from build123d import *

# Parameters (mm, degrees)
BOX001_W               = 70.7107
BOX001_H               = 70.7107
BOX001_DEPTH           = 10
BOX001_PLACEMENT_ANGLE = 315
BOX002_W               = 100
BOX002_H               = 100
BOX002_DEPTH           = 20
BOX_W                  = 200
BOX_H                  = 100
BOX_DEPTH              = 50


with BuildPart() as cube001:
    # Box001 → Box001 (new body)
    with BuildSketch(Plane.XY):
        with Locations((35.35535, 35.35535)):
            Rectangle(BOX001_W, BOX001_H)
    extrude(amount=BOX001_DEPTH)


with BuildPart() as cube001_1:
    # Box001 placement: moved
    add(cube001.part.moved(Location((-50, 0, 40))).rotate(Axis((-50, 0, 40), (0, 0, 1)), BOX001_PLACEMENT_ANGLE))


with BuildPart() as cube002:
    # Box002 → Box002 (new body)
    with BuildSketch(Plane(origin=(0, -50, 10), x_dir=(1, 0, 0), z_dir=(0, 0, 1))):
        with Locations((50, 50)):
            Rectangle(BOX002_W, BOX002_H)
    extrude(amount=BOX002_DEPTH)


with BuildPart() as fusion:
    # Box → Box (new body)
    with BuildSketch(Plane(origin=(0, 50, 0), x_dir=(-1, 0, 0), z_dir=(0, 0, 1))):
        with Locations((100, 50)):
            Rectangle(BOX_W, BOX_H)
    extrude(amount=BOX_DEPTH)

    # Fusion: union Cube001, Cube002
    add(cube001_1.part)
    add(cube002.part)


solid = fusion.part
Model file for the job. Use its own axes, mm. A direction names the side the tool comes from. Give positions to 0.01 mm unless a question says otherwise; leave off trailing zeros. Loops run counter-clockwise (first coordinate to the right, second up) from the corner with the lowest first, then second, coordinate; pieces in that order, holes last. Notation, with made-up numbers: (87.25, 19.25) -> (123.25, 19.25) arc R37 ccw to (123.25, 57.25) -> close; hole circle Ø10 at (-24.5, -28). An arc over 180 degrees is marked (long way). Use a Markdown table: item, result. Add a question column.
(1) Slice it at C-C on x = 56.5. List the corners of the cut face in (y, z).
(2) Wall check: line 1 along Z through (x, y) = (25, 16); line 2 along X through (y, z) = (3, 6); line 3 along Z through (x, y) = (83.5, -26). Give the ranges that are in metal, low to high.
(3) Mould opens along Z. For faces 1 (the flat face through (49, 1, 10)), 2 (the flat face through (100, -1, 20)), 3 (the flat face through (0, 1, 35)) say: +Z half, -Z half, draft (parallel to the pull), parting line (faces both ways), or undercut.
(4) Slice it at A-A on x = 22.5. List the corners of the cut face in (y, z).
(5) Slice it at D-D on y = -7. List the corners of the cut face in (x, z).
(6) Slice it at B-B on y = 6.5. List the corners of the cut face in (x, z), and give its area (3 significant figures).
(7) Drop flat-ended pins along their axis: pin 1 Ø5 at (y, z) = (-0.5, 37) entering from +X; pin 2 Ø1 at (x, y) = (44, 18) entering from +Z; pin 3 Ø15 at (x, y) = (15, 4) entering from -Z. Give the stop position or say it passes through.
(8) Tool access for faces 4 (the flat face through (49, 1, 30)), 5 (the flat face through (0, 1, 5)), 6 (the flat face through (25, -25, 45)): list every direction of +Z, -Z, +X, -X, +Y, -Y with a clear straight run to the whole face (end or side of a thin tool).
Filled sheet:
| question | item | result |
|---|---|---|
| 1 | outline | (-50, 10) -> (50, 10) -> (50, 30) -> (-50, 30) -> close |
| 2 | line 1 | 10 to 30, 40 to 50 |
| 2 | line 2 | -200 to 0 |
| 2 | line 3 | 10 to 30 |
| 3 | face 1 | -Z half |
| 3 | face 2 | draft |
| 3 | face 3 | undercut |
| 4 | outline | (-50, 10) -> (50, 10) -> (50, 30) -> (-50, 30) -> close; (-27.5, 40) -> (27.5, 40) -> (27.5, 50) -> (-27.5, 50) -> close |
| 5 | outline | (-200, 0) -> (0, 0) -> (0, 10) -> (100, 10) -> (100, 30) -> (0, 30) -> (0, 40) -> (43, 40) -> (43, 50) -> (-200, 50) -> close |
| 6 | outline | (-200, 0) -> (0, 0) -> (0, 10) -> (100, 10) -> (100, 30) -> (0, 30) -> (0, 40) -> (43.5, 40) -> (43.5, 50) -> (-200, 50) -> close |
| 6 | area | 12,400 mm2 |
| 7 | pin 1 | x = 0 |
| 7 | pin 2 | z = 30 |
| 7 | pin 3 | z = 10 |
| 8 | face 4 | +X, +Y, -Y |
| 8 | face 5 | -Z, +X, +Y, -Y |
| 8 | face 6 | +Z, +X, -Y |
